Check sheet for the modelled part. Datum: model origin and axes. Units: mm. Face numbers are marked on the shaded views. A direction names the side the tool comes from. Coordinates: 2 decimals unless noted, no trailing zeros. Loops run counter-clockwise (first coordinate to the right, second up) from the corner with the lowest first, then second, coordinate; pieces in that order, holes last. Notation, with made-up numbers: M 17,18 L 62,18 A18 cw 62,25 Z; hole C 70.5,37 d10. An arc over 180 degrees is marked long. Answer in a Markdown table with one row per item. Add a question column.
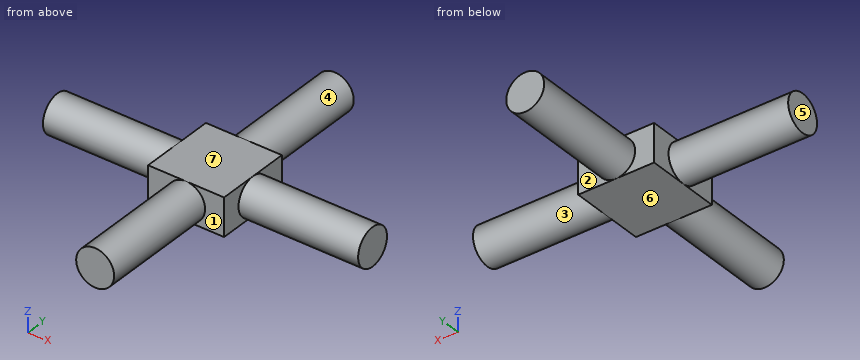
Autodesk Inventor part; units mm, degrees
ref_plane "YZ Plane" through (0, 0, 0) normal (1, 0, 0) x (0, 1, 0)
ref_plane "XZ Plane" through (0, 0, 0) normal (0, 1, 0) x (-1, 0, 0)
ref_plane "XY Plane" through (0, 0, 0) normal (0, 0, 1) x (1, 0, 0)
sketch "Sketch1" plane through (0, 0, 0) normal (0, 1, 0) x (-1, 0, 0)
  line L0 (0, 0) -> (-10, 0) construction
  line L1 (-10, 0) -> (-10, -10)
  line L2 (-10, -10) -> (0, -10)
  line L3 (0, -10) -> (0, 0) construction
  line L4 (-10, 0) -> (-10, 10)
  line L5 (-10, 10) -> (0, 10)
  line L6 (10, 0) -> (10, -10)
  line L7 (10, -10) -> (0, -10)
  line L8 (10, 10) -> (0, 10)
  line L9 (10, 0) -> (10, 10)
  dimension "d0" = 10
extrude "Extrusion1" add sketch "Sketch1" along normal mid plane 10
sketch "Sketch2" plane through (-10, 5, 10) normal (0, 0, 1) x (1, 0, 0)
  circle A0 centre (10, -5) radius 5
  dimension "d4" = 10
extrude "Extrusion2" add sketch "Sketch2" along normal blind 31.5
mirror "Mirror1" about plane through (0, 0, 0) normal (0, 0, 1) of "Extrusion2"
sketch "Sketch3" plane through (10, -5, -10) normal (1, 0, 0) x (0, 0, -1)
  circle A0 centre (-10, 5) radius 5
  dimension "d8" = 10
extrude "Extrusion3" add sketch "Sketch3" along normal blind 31.5
mirror "Mirror2" about plane through (0, 0, 0) normal (1, 0, 0) of "Extrusion3"
move or copy body "Move Body1" bodies to move or copy 1 copy no rotation origin (0, 0, 0) rotation axis (1, 0, 0) rotation angle 90
move or copy body "Move Body2" bodies to move or copy 1 copy no rotation origin (0, 0, 0) rotation axis (0, 0, 1) rotation angle 90
properties part number "HipRoll_v2"
Q1. Access from +Z, -Z, +X, -X, +Y, -Y to the whole of each face (thin tool, end or side, straight path). Record for the marked faces 1, 2 and 3.
Q2. Mould release check, pull along Z, two halves, no side actions. Record for the marked faces 4, 5, 6 and 7: released by +Z, released by -Z, zero draft, split by the parting line, or undercut.
Q3. Thickness scan on L1, parallel to Y at x = -9.5, z = 4; L2, parallel to Y at x = -27, z = 0. Record the ranges inside material, lowest first.
Q4. Cross-section at A-A (z = -3). Record the cut outline in (x, y).
Q5. Cross-section at C-C (y = -7.5). Record the cut outline in (x, z), plus the area to 3 significant figures.
Q6. Go/stop test with flat-tipped pins: pin 1 (2 mm diameter, centred on y = -18.5, z = -2, fed in from -X); pin 2 (1 mm diameter, centred on y = -30.5, z = -4, fed in from +X); pin 3 (1 mm diameter, centred on x = 15, z = 3.5, fed in from -Y). Record where each tip stops, or that it passes through.
Q7. Cross-section at B-B (x = 4). Record the cut outline in (y, z), plus the area to 3 significant figures.
Q8. Cross-section at D-D (z = 2.25). Record the cut outline in (x, y), plus the area to 3 significant figures.
Answer key:
| question | item | result |
|---|---|---|
| 1 | face 1 | +X, -Y |
| 1 | face 2 | +X, +Y |
| 1 | face 3 | +X |
| 2 | face 4 | split by the parting line |
| 2 | face 5 | zero draft |
| 2 | face 6 | released by -Z |
| 2 | face 7 | released by +Z |
| 3 | L1 | -10 to 10 |
| 3 | L2 | -5 to 5 |
| 4 | outline | M -41.5,-4 L -10,-4 L -10,-10 L -4,-10 L -4,-41.5 L 4,-41.5 L 4,-10 L 10,-10 L 10,-4 L 41.5,-4 L 41.5,4 L 10,4 L 10,10 L 4,10 L 4,41.5 L -4,41.5 L -4,10 L -10,10 L -10,4 L -41.5,4 Z |
| 5 | outline | M -10,-5 L 10,-5 L 10,5 L -10,5 Z |
| 5 | area | 200 mm^2 |
| 6 | pin 1 | x = -4.9 |
| 6 | pin 2 | x = 3.57 |
| 6 | pin 3 | y = -4 |
| 7 | outline | M -41.5,-3 L -10,-3 L -10,-5 L 10,-5 L 10,-3 L 41.5,-3 L 41.5,3 L 10,3 L 10,5 L -10,5 L -10,3 L -41.5,3 Z |
| 7 | area | 578 mm^2 |
| 8 | outline | M -41.5,-4.47 L -10,-4.47 L -10,-10 L -4.47,-10 L -4.47,-41.5 L 4.47,-41.5 L 4.47,-10 L 10,-10 L 10,-4.47 L 41.5,-4.47 L 41.5,4.47 L 10,4.47 L 10,10 L 4.47,10 L 4.47,41.5 L -4.47,41.5 L -4.47,10 L -10,10 L -10,4.47 L -41.5,4.47 Z |
| 8 | area | 1,530 mm^2 |
